Part model, mm, in its own coordinate system. Face numbers are marked on the shaded views. A direction names the side the tool comes from. Give positions to 0.01 mm unless a question says otherwise; leave off trailing zeros. Write each loop counter-clockwise with the first axis right and the second up, starting at its lowest first coordinate (ties: lowest second). Pieces come first, ordered by that corner, then holes. Notation, with made-up numbers: M -17,44 L 37,44 A18 cw 37,69 Z; hole C 6,67 d3. An arc over 180 degrees is marked long. Use CSV: the item, a comma, the result in double quotes. Start each with the question number.
1. Band-saw the part on A-A, the plane x = -30.5. List the corners of the cut face in (y, z), then the cut area to 3 significant figures.
2. Mould opens along Y. For the marked faces 1, 2 and 3 say: pulls with the +Y half, pulls with the -Y half, needs draft (parallel to the pull), parting line crosses it, or undercut.
3. Band-saw the part on D-D, the plane z = 7.5. List the corners of the cut face in (x, y), then the cut area to 3 significant figures.
4. Band-saw the part on C-C, the plane z = 43. List the corners of the cut face in (x, y).
5. 3-axis set-ups, long thin cutter, end or side, ignore diameter. For the marked faces 4, 5 and 6: which of +Z, -Z, +X, -X, +Y, -Y reach the whole face in a straight line?
6. Drill centre lines: line 1 along X through (y, z) = (29, 38); line 2 along Y through (x, z) = (-11, 3.5); line 3 along Z through (x, y) = (34.5, -29). Where is each one in solid material? Low to high. Write a range as from..to.
7. Band-saw the part on B-B, the plane y = -23. List the corners of the cut face in (x, z).
8. Drop flat-ended pins along their axis: pin 1 Ø25 at (x, y) = (-7, 32.5) entering from -Z; pin 2 Ø8 at (x, y) = (-3, -58) entering from +Z; pin 3 Ø0.6 at (x, y) = (39.5, -16) entering from -Z. Give the stop position or say it passes through.
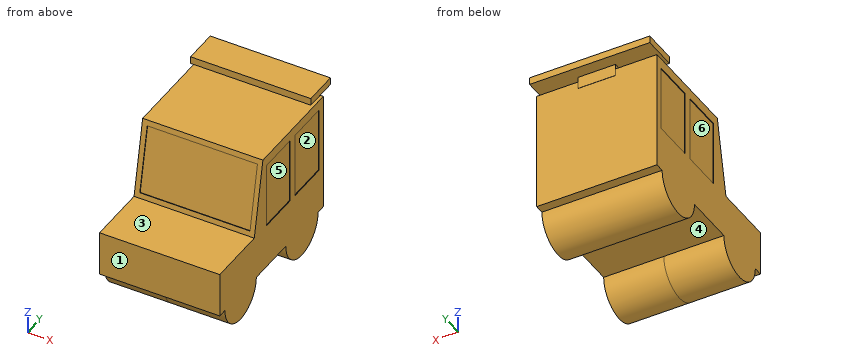
from build123d import *

# Parameters (mm, degrees)
F2_DEPTH  = 40
F1_R      = 18.2030638816
F1_R_2    = 18.7046022313
F3_DEPTH  = 40
F4_W      = 27.0581897348
F4_H      = 43.6939634383
F4_W_2    = 27.8599155135
F5_DEPTH  = 0.5
F6_W      = 73.3577571809
F6_H      = 43.7416750938
F7_DEPTH  = 0.5
F8_W      = 7.9477988183
F8_H      = 10.0772306323
F9_DEPTH  = 12.5
F10_W     = 22.8018909693
F10_H     = 4.7676712275
F11_DEPTH = 40


# Not quite as in the source:
# - a pattern or mirror of a feature is missing from the dataset's text; its kind, count and spacing are read off the source's solid
# - a feature names something its author has since deleted; it is built from what else it names


with BuildPart() as f2:
    # F0 (on Right) → F2 (new body, symmetric)
    with BuildSketch(Plane.YZ):
        Polygon((-85.6041714479, 30), (-85.6041714479, 0), (34.3958285521, 0), (34.3958285521, 80), (-35.6041714479, 80), (-45.6041714479, 30), align=None)
    extrude(amount=F2_DEPTH, both=True)

    # F1 (on Right) → F3 (join, symmetric)
    with BuildSketch(Plane.YZ):
        with Locations((-61.4385381341, 0)):
            Circle(F1_R)
        with Locations((9.633612819, 0)):
            Circle(F1_R_2)
    extrude(amount=F3_DEPTH, both=True)

    # F4 (on face) → F5 (cut, symmetric)
    with BuildSketch(Plane.YZ.offset(40)):
        with Locations((-17.7288064733, 51.5053849667)):
            Rectangle(F4_W, F4_H)
        with Locations((15.7431771513, 51.5053849667)):
            Rectangle(F4_W_2, F4_H)
    f5 = extrude(amount=F5_DEPTH, both=True, mode=Mode.SUBTRACT)

    # F5_copies: F5 across plane
    add(f5.mirror(Plane(origin=(0, 0, 0), x_dir=(0, 0, -1), z_dir=(-1, 0, 0))), mode=Mode.SUBTRACT)

    # F6 (on face) → F7 (cut, symmetric)
    with BuildSketch(Plane(origin=(0, -49.619395623, 9.9238791246), x_dir=(1, 0, 0), z_dir=(0, -0.9805806757, 0.1961161351))):
        with Locations((0.100215897, 45.8797877654)):
            Rectangle(F6_W, F6_H)
    extrude(amount=F7_DEPTH, both=True, mode=Mode.SUBTRACT)

    # F8 (on Right) → F9 (join, symmetric)
    with BuildSketch(Plane.YZ):
        with Locations((30.565129593, 80.2655704319)):
            Rectangle(F8_W, F8_H)
    extrude(amount=F9_DEPTH, both=True)

    # F10 (on Right) → F11 (join, symmetric)
    with BuildSketch(Plane.YZ):
        with Locations((31.2845855951, 85.5805724859)):
            Rectangle(F10_W, F10_H)
    extrude(amount=F11_DEPTH, both=True)


solid = f2.part
Output:
1,outline,"M -85.6,0 L -79.64,0 A18.2 ccw -43.24,0 L -9.07,0 A18.7 ccw 28.34,0 L 34.4,0 L 34.4,80 L -35.6,80 L -36.33,76.36 L -35.84,76.26 L -44.42,33.37 L -44.91,33.47 L -45.6,30 L -85.6,30 Z; M 19.88,83.2 L 42.69,83.2 L 42.69,87.96 L 19.88,87.96 Z"
1,area,"8,510 mm²"
2,face 1,"pulls with the -Y half"
2,face 2,"undercut"
2,face 3,"needs draft"
3,outline,"M -40,-85.6 L 40,-85.6 L 40,34.4 L -40,34.4 Z"
3,area,"9,600 mm²"
4,outline,"M -40,-43 L -36.58,-43 L -36.58,-42.49 L 36.78,-42.49 L 36.78,-43 L 40,-43 L 40,-31.26 L 39.5,-31.26 L 39.5,-4.2 L 40,-4.2 L 40,1.81 L 39.5,1.81 L 39.5,29.67 L 40,29.67 L 40,34.4 L -40,34.4 L -40,29.67 L -39.5,29.67 L -39.5,1.81 L -40,1.81 L -40,-4.2 L -39.5,-4.2 L -39.5,-31.26 L -40,-31.26 Z"
5,face 4,"-Z, +X, -X"
5,face 5,"+X"
5,face 6,"-X"
6,line 1,"x = -39.5..39.5"
6,line 2,"y = -85.6..34.4"
6,line 3,"z = 0..80"
7,outline,"M -40,0 L 40,0 L 40,29.66 L 39.5,29.66 L 39.5,73.35 L 40,73.35 L 40,80 L -40,80 L -40,73.35 L -39.5,73.35 L -39.5,29.66 L -40,29.66 Z"
8,pin 1,"stops at z = -15.57"
8,pin 2,"stops at z = 30"
8,pin 3,"stops at z = 0"
